Verification items for the finished model (mm, model axes). Face numbers are marked on the shaded views. A direction names the side the tool comes from. Coordinates: 2 decimals unless noted, no trailing zeros. Write each loop counter-clockwise with the first axis right and the second up, starting at its lowest first coordinate (ties: lowest second). Pieces come first, ordered by that corner, then holes. Notation, with made-up numbers: (-1.75, 26) -> (52.25, 26) arc R34 ccw to (52.25, 57) -> close; hole circle Ø1 at (-34.75, 53.5). An arc over 180 degrees is marked (long way). Use a Markdown table: item, result. Add a question column.
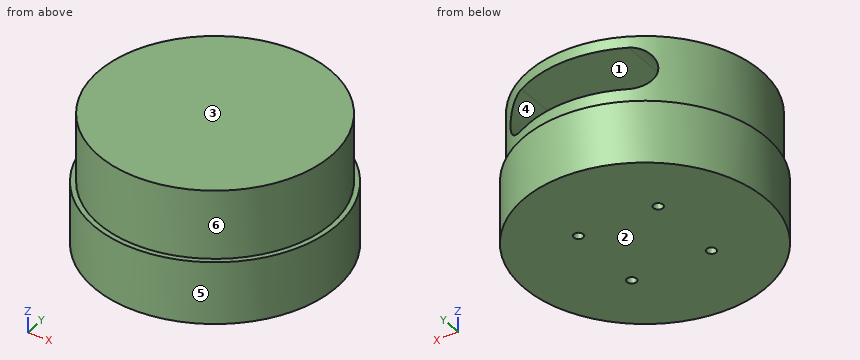
from build123d import *

# Parameters (mm, degrees)
SKETCH_R           = 37.85
PAD_DEPTH          = 19.4
SKETCH001_R        = 36.25
PAD001_DEPTH       = 21.4
POCKET_DEPTH       = 50
SKETCH003_R        = 1.5
POCKET001_DEPTH    = 5
POLARPATTERN_COUNT = 4


with BuildPart() as part:
    # Sketch → Pad (new body)
    with BuildSketch(Plane.XY):
        Circle(SKETCH_R)
    extrude(amount=PAD_DEPTH)

    # Sketch001 (on Face3 of Pad) → Pad001 (join)
    with BuildSketch(Plane.XY.offset(19.4)):
        Circle(SKETCH001_R)
    extrude(amount=PAD001_DEPTH)

    # Sketch002 → Pocket (cut)
    with BuildSketch(Plane.XZ):
        with BuildLine():
            ThreePointArc((-16.437559, 37.3), (-22.937559, 30.8), (-16.437559, 24.3))
            Line((-16.437559, 24.3), (17.562441, 24.3))
            ThreePointArc((17.562441, 24.3), (24.062441, 30.8), (17.562441, 37.3))
            Line((-16.437559, 37.3), (17.562441, 37.3))
        make_face()
    extrude(amount=-POCKET_DEPTH, mode=Mode.SUBTRACT)

    # Sketch003 (on Face2 of Pocket) → Pocket001 (cut)
    with BuildSketch(Plane(origin=(0, 0, 0), x_dir=(1, 0, 0), z_dir=(0, 0, -1))):
        with Locations((-12.5, 12.5)):
            Circle(SKETCH003_R)
    pocket001 = extrude(amount=-POCKET001_DEPTH, mode=Mode.SUBTRACT)

    # PolarPattern: Pocket001 ×4 about axis
    polarpattern_axis = Axis((0, 0, 0), (0, 0, -1))
    for i in range(1, POLARPATTERN_COUNT):
        add(pocket001.rotate(polarpattern_axis, i * 360 / POLARPATTERN_COUNT), mode=Mode.SUBTRACT)


solid = part.part
1) Cross-section at A-A on z = 4. Record the boundary of the cut face in (x, y).
2) Cross-section at D-D on y = -12.5. Record the boundary of the cut face in (x, z).
3) Gauge pin test, flat ends, axial feed: pin 1 (3 mm diameter, centred on y = -26, z = 18.5, fed in from +X); pin 2 (4 mm diameter, centred on y = -29, z = 23, fed in from +X); pin 3 (10 mm diameter, centred on x = -22.5, z = 5, fed in from -Y). Record the tip position at first contact, or that the pin passes through.
4) Set-up check for the marked faces 4, 5 and 6: record each of +Z, -Z, +X, -X, +Y, -Y from which the full face is reachable in a straight line by a thin tool's end or side.
5) Cross-section at B-B on y = 19.5. Record the boundary of the cut face in (x, z), then the cut area to 3 significant figures.
6) Release check for a two-part mould opening along Z. For the marked faces 1, 2 and 3 record: released by +Z, released by -Z, zero draft, split by the parting line, or undercut.
7) Thickness scan on L1, parallel to Y at x = -12.5, z = 1.75; L2, parallel to X at y = -12, z = 2. Record the ranges inside material, lowest first.
8) Cross-section at C-C on x = 0. Record the boundary of the cut face in (y, z).
Returned:
| question | item | result |
|---|---|---|
| 1 | outline | circle Ø75.7 at (0, 0); hole circle Ø3 at (-12.5, -12.5); hole circle Ø3 at (-12.5, 12.5); hole circle Ø3 at (12.5, -12.5); hole circle Ø3 at (12.5, 12.5) |
| 2 | outline | (-35.73, 0) -> (-14, 0) -> (-14, 5) -> (-11, 5) -> (-11, 0) -> (11, 0) -> (11, 5) -> (14, 5) -> (14, 0) -> (35.73, 0) -> (35.73, 19.4) -> (34.03, 19.4) -> (34.03, 40.8) -> (-34.03, 40.8) -> (-34.03, 19.4) -> (-35.73, 19.4) -> close |
| 3 | pin 1 | stops at x = 28.85 |
| 3 | pin 2 | stops at x = 24.19 |
| 3 | pin 3 | stops at y = -33.56 |
| 4 | face 4 | +Y |
| 4 | face 5 | +Z, -Z |
| 4 | face 6 | +Z |
| 5 | outline | (-32.44, 0) -> (32.44, 0) -> (32.44, 19.4) -> (30.56, 19.4) -> (30.56, 40.8) -> (-30.56, 40.8) -> (-30.56, 19.4) -> (-32.44, 19.4) -> close; hole (-16.44, 24.3) -> (17.56, 24.3) arc R6.5 ccw to (17.56, 37.3) -> (-16.44, 37.3) arc R6.5 ccw to start |
| 5 | area | 1,990 mm² |
| 6 | face 1 | undercut |
| 6 | face 2 | released by -Z |
| 6 | face 3 | released by +Z |
| 7 | L1 | y = -35.73 to -14, -11 to 11, 14 to 35.73 |
| 7 | L2 | x = -35.9 to -13.91, -11.09 to 11.09, 13.91 to 35.9 |
| 8 | outline | (-37.85, 0) -> (37.85, 0) -> (37.85, 19.4) -> (36.25, 19.4) -> (36.25, 24.3) -> (0, 24.3) -> (0, 37.3) -> (36.25, 37.3) -> (36.25, 40.8) -> (-36.25, 40.8) -> (-36.25, 19.4) -> (-37.85, 19.4) -> close |
